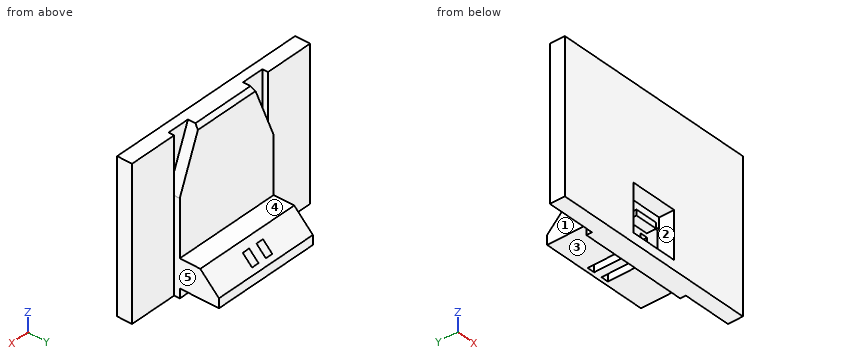
from build123d import *

# Parameters (mm, degrees)
SKETCH_1_W          = 110
SKETCH_1_H          = 80
EXTRUDE_1_DEPTH     = 8
SKETCH_3_W          = 58
SKETCH_3_H          = 80
EXTRUDE_2_DEPTH     = 9
CUT_EXTRUDE_2_DEPTH = 6
CHAMFER_5_SIZE      = 2
SKETCH_10_W         = 58
SKETCH_10_H         = 15
EXTRUDE_5_DEPTH     = 30
CHAMFER_9_SIZE      = 10
SKETCH_11_W         = 4
SKETCH_11_H         = 12
CUT_EXTRUDE_6_DEPTH = 30
SKETCH_12_W         = 25
SKETCH_12_H         = 25
CUT_EXTRUDE_7_DEPTH = 9
SKETCH_13_W         = 12
SKETCH_13_H         = 3
EXTRUDE_6_DEPTH     = 5
SKETCH_14_W         = 25
SKETCH_14_H         = 5.959996218
EXTRUDE_7_DEPTH     = 1


with BuildPart() as part:
    # 草图1 → 凸台-拉伸1 (new body)
    with BuildSketch(Plane(origin=(0, 0, 0), x_dir=(1, 0, 0), z_dir=(0, 1, 0))):
        Rectangle(SKETCH_1_W, SKETCH_1_H)
    extrude(amount=EXTRUDE_1_DEPTH)

    # 草图3 → 凸台-拉伸2 (add)
    with BuildSketch(Plane(origin=(0, 2, 0), x_dir=(1, 0, 0), z_dir=(0, 1, 0))):
        Rectangle(SKETCH_3_W, SKETCH_3_H)
    extrude(amount=EXTRUDE_2_DEPTH)

    # 草图4 → 切除-拉伸2 (cut)
    with BuildSketch(Plane(origin=(0, 11, 0), x_dir=(1, 0, 0), z_dir=(0, 1, 0))):
        Polygon((-29, -10), (-29, -40), (-17, -40), align=None)
        Polygon((17, -40), (29, -10), (29, -40), align=None)
    extrude(amount=-CUT_EXTRUDE_2_DEPTH, mode=Mode.SUBTRACT)

    # 倒角5
    chamfer_5_edges = [part.edges().sort_by_distance(p)[0] for p in [
        (0, 11, 40),
    ]]
    chamfer(chamfer_5_edges, length=CHAMFER_5_SIZE)

    # 草图10 → 凸台-拉伸5 (add)
    with BuildSketch(Plane(origin=(0, 2, 0), x_dir=(1, 0, 0), z_dir=(0, 1, 0))):
        with Locations((0, 27.5)):
            Rectangle(SKETCH_10_W, SKETCH_10_H)
    extrude(amount=EXTRUDE_5_DEPTH)

    # 倒角9
    chamfer_9_edges = [part.edges().sort_by_distance(p)[0] for p in [
        (0, 32, -20),
    ]]
    chamfer(chamfer_9_edges, length=CHAMFER_9_SIZE)

    # 草图11 → 切除-拉伸6 (cut)
    with BuildSketch(Plane.XZ):
        with Locations((-4.25, -29)):
            Rectangle(SKETCH_11_W, SKETCH_11_H)
        with Locations((4.25, -29)):
            Rectangle(SKETCH_11_W, SKETCH_11_H)
    extrude(amount=-CUT_EXTRUDE_6_DEPTH, mode=Mode.SUBTRACT)

    # 草图12 → 切除-拉伸7 (cut)
    with BuildSketch(Plane.XZ):
        with Locations((0, -22.5)):
            Rectangle(SKETCH_12_W, SKETCH_12_H)
    extrude(amount=-CUT_EXTRUDE_7_DEPTH, mode=Mode.SUBTRACT)

    # 草图13 → 凸台-拉伸6 (add)
    with BuildSketch(Plane.XZ.offset(-9)):
        with Locations((0, -19.5)):
            Rectangle(SKETCH_13_W, SKETCH_13_H)
    extrude(amount=EXTRUDE_6_DEPTH)

    # 草图14 → 凸台-拉伸7 (add)
    with BuildSketch(Plane.XZ.offset(-9)):
        with Locations((0, -12.979998109)):
            Rectangle(SKETCH_14_W, SKETCH_14_H)
    extrude(amount=EXTRUDE_7_DEPTH)


solid = part.part
Read the model definition and answer for the solid it produces. Units are mm, in the model's axes. Face numbers are marked on the shaded views. A direction names the side the tool comes from. Give positions to 0.01 mm unless a question says otherwise; leave off trailing zeros. Write each loop counter-clockwise with the first axis right and the second up, starting at its lowest first coordinate (ties: lowest second). Pieces come first, ordered by that corner, then holes. Notation, with made-up numbers: (36, -3) -> (89, -3) arc R20 ccw to (89, 23) -> close; hole circle Ø6 at (33.25, -33.5). An arc over 180 degrees is marked (long way). Answer as a JSON object with one key per item and string values. Group by question number.
1) Find section C-C (x = -27.5). Write down the section's boundary in (y, z).
2) Find section D-D (y = 17). Write down the section's boundary in (x, z).
3) Find section B-B (z = -3). Write down the section's boundary in (x, y), and give its area (3 significant figures).
4) Consider L1, parallel to X at y = 29, z = -27.5; L2, parallel to Z at x = -11.5, y = 6; L3, parallel to Y at x = -4.5, z = 37. Determine where each line is inside the solid, lowest interval first. Write a range as from..to.
5) Find section A-A (y = 28). Write down the section's boundary in (x, z).
6) A tool of negligible diameter and unlimited length cuts with its end or side. For the marked faces 1, 2, 3, 4 and 5, from which of +Z, -Z, +X, -X, +Y, -Y can it reach the whole face along a straight path? Write none if from no direction.
7) Each of these flat-tipped pins is pushed along its axis until it touches: P1, Ø5, axis at x = -20, y = 27, coming from the -Z side; P2, Ø5, axis at x = -20, y = 27.5, coming from the +Z side; P3, Ø13, axis at y = 21, z = -27, coming from the -X side; P4, Ø4, axis at x = -11, z = -1.5, coming from the -Y side. Where does it stop, or does it pass through?
Values follow:
{
 "1": {"outline": "(0, -40) -> (11, -40) -> (11, -35) -> (32, -35) -> (32, -30) -> (22, -20) -> (11, -20) -> (11, 13.75) -> (5, 13.75) -> (5, 40) -> (0, 40) -> close"},
 "2": {"outline": "(-29, -35) -> (-6.25, -35) -> (-6.25, -23) -> (-2.25, -23) -> (-2.25, -35) -> (2.25, -35) -> (2.25, -23) -> (6.25, -23) -> (6.25, -35) -> (29, -35) -> (29, -20) -> (-29, -20) -> close"},
 "3": {"outline": "(-55, 0) -> (55, 0) -> (55, 8) -> (29, 8) -> (29, 11) -> (-29, 11) -> (-29, 8) -> (-55, 8) -> close", "area": "1,050 mm2"},
 "4": {"L1": "x = -29..-6.25, -2.25..2.25, 6.25..29", "L2": "z = -40..-35, -10..40", "L3": "y = 0..11"},
 "5": {"outline": "(-29, -35) -> (-6.25, -35) -> (-6.25, -26) -> (-29, -26) -> close; (-2.25, -35) -> (2.25, -35) -> (2.25, -26) -> (-2.25, -26) -> close; (6.25, -35) -> (29, -35) -> (29, -26) -> (6.25, -26) -> close"},
 "6": {"face 1": "+Z, -Z, -X, +Y", "face 2": "-Y", "face 3": "-Z, +X, -X, +Y", "face 4": "+Z, +X, -X, +Y", "face 5": "+Z, -Z, +X, +Y"},
 "7": {"P1": "stops at z = -35", "P2": "stops at z = -23", "P3": "stops at x = -29", "P4": "stops at y = 0"}
}
